Part model, mm, in its own coordinate system. Give positions to 0.01 mm unless a question says otherwise; leave off trailing zeros. Order: outer loops, then holes, each group sorted by start corner. A loop starts at its lowest first (then second) coordinate and runs counter-clockwise, first axis right, second up. Notation, with made-up numbers: (-2, 32.25) - (15, 32.25) arc R23 cw to (15, 70.25) - close; hole circle Ø2 at (23, 49.25). An arc over 180 degrees is marked (long way). One line per item, written item: value.
```python
from build123d import *

# Parameters (mm, degrees)
SKETCH1_W           = 765
SKETCH1_H           = 765
BOSS_EXTRUDE1_DEPTH = 16
CUT_EXTRUDE2_REACH  = 18
SKETCH5_R           = 50


with BuildPart() as part:
    # Sketch1 → Boss-Extrude1 (new body)
    with BuildSketch(Plane(origin=(0, 0, 0), x_dir=(1, 0, 0), z_dir=(0, 1, 0))):
        Rectangle(SKETCH1_W, SKETCH1_H)
    extrude(amount=BOSS_EXTRUDE1_DEPTH)

    # Sketch5 → Cut-Extrude2 (cut, up to next)
    with BuildSketch(Plane(origin=(0, 16, 0), x_dir=(1, 0, 0), z_dir=(0, 1, 0)), mode=Mode.PRIVATE) as cut_extrude2_sk1:
        with Locations((-250, 250)):
            Circle(SKETCH5_R)
    cut_extrude2_tool1 = extrude(cut_extrude2_sk1.sketch, amount=-CUT_EXTRUDE2_REACH, mode=Mode.PRIVATE) & part.part
    add(cut_extrude2_tool1.solids().sort_by_distance((-250, 16, -250))[0], mode=Mode.SUBTRACT)
    # Sketch5 → Cut-Extrude2 (cut, up to next)
    with BuildSketch(Plane(origin=(0, 16, 0), x_dir=(1, 0, 0), z_dir=(0, 1, 0)), mode=Mode.PRIVATE) as cut_extrude2_sk2:
        with Locations((250, 250)):
            Circle(SKETCH5_R)
    cut_extrude2_tool2 = extrude(cut_extrude2_sk2.sketch, amount=-CUT_EXTRUDE2_REACH, mode=Mode.PRIVATE) & part.part
    add(cut_extrude2_tool2.solids().sort_by_distance((250, 16, -250))[0], mode=Mode.SUBTRACT)
    # Sketch5 → Cut-Extrude2 (cut, up to next)
    with BuildSketch(Plane(origin=(0, 16, 0), x_dir=(1, 0, 0), z_dir=(0, 1, 0)), mode=Mode.PRIVATE) as cut_extrude2_sk3:
        with Locations((250, -250)):
            Circle(SKETCH5_R)
    cut_extrude2_tool3 = extrude(cut_extrude2_sk3.sketch, amount=-CUT_EXTRUDE2_REACH, mode=Mode.PRIVATE) & part.part
    add(cut_extrude2_tool3.solids().sort_by_distance((250, 16, 250))[0], mode=Mode.SUBTRACT)
    # Sketch5 → Cut-Extrude2 (cut, up to next)
    with BuildSketch(Plane(origin=(0, 16, 0), x_dir=(1, 0, 0), z_dir=(0, 1, 0)), mode=Mode.PRIVATE) as cut_extrude2_sk4:
        with Locations((-250, -250)):
            Circle(SKETCH5_R)
    cut_extrude2_tool4 = extrude(cut_extrude2_sk4.sketch, amount=-CUT_EXTRUDE2_REACH, mode=Mode.PRIVATE) & part.part
    add(cut_extrude2_tool4.solids().sort_by_distance((-250, 16, 250))[0], mode=Mode.SUBTRACT)


solid = part.part
```
1) Slice it at C-C on y = 10. Write the cut outline in (x, z).
Answer:
outline: (-382.5, -382.5) - (382.5, -382.5) - (382.5, 382.5) - (-382.5, 382.5) - close; hole circle Ø100 at (-250, -250); hole circle Ø100 at (-250, 250); hole circle Ø100 at (250, -250); hole circle Ø100 at (250, 250)
2) Wall check: line 1 along Z through (x, y) = (250, 4.5); line 2 along X through (y, z) = (1.75, -284.5). Give the ranges that are in metal, low to high. Write a range as [from, to].
Answer:
line 1: z = [-382.5, -300], [-200, 200], [300, 382.5]
line 2: x = [-382.5, -286.19], [-213.81, 213.81], [286.19, 382.5]
3) Slice it at B-B on x = -250. Write the cut outline in (y, z), then the cut area to 3 significant figures.
Answer:
outline: (0, -382.5) - (16, -382.5) - (16, -300) - (0, -300) - close; (0, -200) - (16, -200) - (16, 200) - (0, 200) - close; (0, 300) - (16, 300) - (16, 382.5) - (0, 382.5) - close
area: 9,040 mm2
4) Slice it at A-A on z = -250. Write the cut outline in (x, y).
Answer:
outline: (-382.5, 0) - (-300, 0) - (-300, 16) - (-382.5, 16) - close; (-200, 0) - (200, 0) - (200, 16) - (-200, 16) - close; (300, 0) - (382.5, 0) - (382.5, 16) - (300, 16) - close
5) Drop a flat-ended pin along its axis: P1, Ø1.5, axis at x = -143, z = -195.5, coming from the -Y side. Give the stop position or say it passes through.
Answer:
P1: stops at y = 0
6) Two-plate mould, pull along Z, no slides. Class faces 1 (the face through (-256.509, 8.112, -299.575)), 2 (the face through (-5, 16, -5)): pulls with the +Z half, pulls with the -Z half, needs draft (parallel to the pull), parting line crosses it, or undercut.
Answer:
face 1: undercut
face 2: needs draft
